Check sheet for the modelled part. Datum: model origin and axes. Units: mm. Give positions to 0.01 mm unless a question says otherwise; leave off trailing zeros. Write each loop counter-clockwise with the first axis right and the second up, starting at its lowest first coordinate (ties: lowest second). Pieces come first, ordered by that corner, then holes. Notation, with made-up numbers: (23, -25) -> (28, -25) arc R21 cw to (28, -7) -> close; hole circle Ø5 at (67.25, 84.5). An arc over 180 degrees is marked (long way). Use a Markdown table: item, result. Add a question column.
1. Release check for a two-part mould opening along Y. For faces 1 (the cylindrical face through (0, -1, -11)), 2 (the flat face through (0, 0, -21.2)), 3 (the flat face through (0, 0, -1)) record: released by +Y, released by -Y, zero draft, split by the parting line, or undercut.
2. Scan lines: probe 1 along X at (y, z) = (-0.8, -7.75); probe 2 along X at (y, z) = (-0.6, -9). Record each from-to range of solid material in increasing order. Write a range as [from, to].
3. Cross-section at A-A (z = -5.25). Enter the section's corners in (x, y), then the cut area to 3 significant figures.
Autodesk Inventor part; units mm, degrees
ref_plane "YZ Plane" through (0, 0, 0) normal (1, 0, 0) x (0, 1, 0)
ref_plane "XZ Plane" through (0, 0, 0) normal (0, 1, 0) x (-1, 0, 0)
ref_plane "XY Plane" through (0, 0, 0) normal (0, 0, 1) x (1, 0, 0)
sketch "Sketch2" plane through (0, 0, 0) normal (0, 1, 0) x (-1, 0, 0)
  line L0 (0, 0) -> (1.75, 0)
  line L1 (1.75, 0) -> (1.75, -1.2)
  line L2 (1.75, -1.2) -> (1, -1.2)
  line L3 (1, -1.2) -> (1, -21.2)
  line L4 (1, -21.2) -> (0, -21.2)
  line L5 (0, 0) -> (0, -21.2)
  dimension "d9" = 1.75
  dimension "d10" = 1.2
  dimension "d12" = 20
  dimension "d19" = 2
revolve "Revolution1" add sketch "Sketch2" angle 360 about axis through (0, 0, 0) along (0, 0, -1)
fillet "Fillet1" radius 1 1 edges at (1.75, 0, 0)
chamfer "Chamfer1" distance 0.2 angle 45 1 edges at (1, 0, -21.2)
thread "Thread1"
sketch "Sketch4" plane through (0, 0, 0) normal (0, 0, 1) x (1, 0, 0)
  line L0 (0, 0.5774) -> (0.5, 0.2887)
  line L1 (0.5, 0.2887) -> (0.5, -0.2887)
  line L2 (0.5, -0.2887) -> (0, -0.5774)
  line L3 (0, -0.5774) -> (-0.5, -0.2887)
  line L4 (-0.5, -0.2887) -> (-0.5, 0.2887)
  line L5 (-0.5, 0.2887) -> (0, 0.5774)
  point P0 (0, 0)
  point P1 (0, 0)
  dimension "d22" = 1
  dimension "d24" = 0.2887
extrude "Extrusion2" cut sketch "Sketch4" against normal blind 1
chamfer "Chamfer2" distance 0.1 angle 45 12 edges at (-0.5, 0, 0) (-0.25, 0.433, 0) (0.25, 0.433, 0) (0.5, 0, 0) (0.25, -0.433, 0) (-0.25, -0.433, 0) (-0.25, 0.433, -1) (-0.5, 0, -1) (-0.25, -0.433, -1) (0.25, -0.433, -1) (0.5, 0, -1) (0.25, 0.433, -1)
properties part number "rapoukHexagonScrewM2×20v0" material "Steel, Carbon"
Worked answers:
| question | item | result |
|---|---|---|
| 1 | face 1 | split by the parting line |
| 1 | face 2 | zero draft |
| 1 | face 3 | undercut |
| 2 | probe 1 | x = [-0.6, 0.6] |
| 2 | probe 2 | x = [-0.8, 0.8] |
| 3 | outline | circle Ø2 at (0, 0) |
| 3 | area | 3.14 mm² |
